from build123d import *

# Parameters (mm, degrees)
F1_W     = 940
F1_H     = 760
F1_W_2   = 30
F1_H_2   = 700
F2_DEPTH = 30
F0_R     = 1.4
F0_R_2   = 13
F3_DEPTH = 5
F4_W     = 30
F4_H     = 30
F5_DEPTH = 770


with BuildPart() as f2:
    # F1 (on Top) → F2 (new body)
    with BuildSketch(Plane.XY):
        with Locations((0, -20)):
            Rectangle(F1_W, F1_H)
        Polygon((-440, -370), (-440, 330), (-80, 330), (-50, 330), (50, 330), (80, 330), (440, 330), (440, -370), (80, -370), (50, -370), (-50, -370), (-80, -370), align=None, mode=Mode.SUBTRACT)
        with Locations((-65, -20)):
            Rectangle(F1_W_2, F1_H_2)
        with Locations((65, -20)):
            Rectangle(F1_W_2, F1_H_2)
    extrude(amount=-F2_DEPTH)

    # F0 (on Top) → F3 (join)
    with BuildSketch(Plane.XY):
        with BuildLine():
            Line((-67.5, 150), (-150, 150))
            Line((-150, 150), (-150, -387.5))
            Line((-150, -387.5), (-140, -387.5))
            ThreePointArc((-140, -387.5), (-137.5, -390), (-140, -392.5))
            Line((-140, -392.5), (-150, -392.5))
            Line((-150, -392.5), (-150, -475))
            Line((-150, -475), (-106, -475))
            ThreePointArc((-106, -475), (-93.5, -469), (-81, -475))
            Line((-81, -475), (0, -475))
            Line((0, -475), (81, -475))
            ThreePointArc((81, -475), (93.5, -469), (106, -475))
            Line((106, -475), (150, -475))
            Line((150, -475), (150, -392.5))
            Line((150, -392.5), (140, -392.5))
            ThreePointArc((140, -392.5), (137.5, -390), (140, -387.5))
            Line((140, -387.5), (150, -387.5))
            Line((150, -387.5), (150, 150))
            Line((150, 150), (67.5, 150))
            Line((67.5, 150), (67.5, 140))
            ThreePointArc((67.5, 140), (65, 137.5), (62.5, 140))
            Line((62.5, 140), (62.5, 150))
            Line((62.5, 150), (-62.5, 150))
            Line((-62.5, 150), (-62.5, 140))
            ThreePointArc((-62.5, 140), (-65, 137.5), (-67.5, 140))
            Line((-67.5, 140), (-67.5, 150))
        make_face()
        with Locations((-106, -468)):
            Circle(F0_R, mode=Mode.SUBTRACT)
        with Locations((-81, -468)):
            Circle(F0_R, mode=Mode.SUBTRACT)
        with Locations((81, -468)):
            Circle(F0_R, mode=Mode.SUBTRACT)
        with Locations((106, -468)):
            Circle(F0_R, mode=Mode.SUBTRACT)
        with Locations((-114.904852, -139.653589)):
            Circle(F0_R, mode=Mode.SUBTRACT)
        with Locations((-139.653589, -114.904852)):
            Circle(F0_R, mode=Mode.SUBTRACT)
        with Locations((-139.653589, 114.904852)):
            Circle(F0_R, mode=Mode.SUBTRACT)
        with Locations((-114.904852, 139.653589)):
            Circle(F0_R, mode=Mode.SUBTRACT)
        with Locations((0, -22)):
            Circle(F0_R, mode=Mode.SUBTRACT)
        with Locations((114.904852, -139.653589)):
            Circle(F0_R, mode=Mode.SUBTRACT)
        with Locations((139.653589, -114.904852)):
            Circle(F0_R, mode=Mode.SUBTRACT)
        Circle(F0_R_2, mode=Mode.SUBTRACT)
        with Locations((0, 22)):
            Circle(F0_R, mode=Mode.SUBTRACT)
        with Locations((114.904852, 139.653589)):
            Circle(F0_R, mode=Mode.SUBTRACT)
        with Locations((139.653589, 114.904852)):
            Circle(F0_R, mode=Mode.SUBTRACT)
    extrude(amount=F3_DEPTH)

    # F4 (on face) → F5 (join)
    with BuildSketch(Plane(origin=(0, 0, -30), x_dir=(1, 0, 0), z_dir=(0, 0, -1))):
        with Locations((-455, 385)):
            Rectangle(F4_W, F4_H)
        with Locations((-455, -345)):
            Rectangle(F4_W, F4_H)
        with Locations((455, -345)):
            Rectangle(F4_W, F4_H)
        with Locations((455, 385)):
            Rectangle(F4_W, F4_H)
    extrude(amount=F5_DEPTH)


solid = f2.part
The listing builds one solid part. Answer for the finished solid, in the listing's coordinates (mm). A direction names the side the tool comes from. Round coordinates to 2 decimals unless told otherwise and drop trailing zeros. Order: outer loops, then holes, each group sorted by start corner. A loop starts at its lowest first (then second) coordinate and runs counter-clockwise, first axis right, second up. Notation, with made-up numbers: (-37, 83) -> (-26, 83) arc R17 ccw to (-26, 97) -> close; hole circle Ø2 at (67.5, 89.25). An arc over 180 degrees is marked (long way). Put each result on its own line as item: value.
Q1. Consider line 1 along Y through (x, z) = (0, 3.95); line 2 along X through (y, z) = (-468, 2.1); line 3 along X through (y, z) = (-393.5, -236). Determine where each line is inside the solid, lowest interval first.
Results list:
line 1: -475 to -23.4, -20.6 to -13, 13 to 20.6, 23.4 to 150
line 2: -150 to -107.4, -104.6 to -82.4, -79.6 to 79.6, 82.4 to 104.6, 107.4 to 150
line 3: -470 to -440, 440 to 470
Q2. Section A-A, the plane y = 44 is taken. Write down the section's boundary in (x, z).
Results list:
outline: (-470, -30) -> (-440, -30) -> (-440, 0) -> (-470, 0) -> close; (-150, 0) -> (-80, 0) -> (-80, -30) -> (-50, -30) -> (-50, 0) -> (50, 0) -> (50, -30) -> (80, -30) -> (80, 0) -> (150, 0) -> (150, 5) -> (-150, 5) -> close; (440, -30) -> (470, -30) -> (470, 0) -> (440, 0) -> close
Q3. Section D-D, the plane y = 273.5 is taken. Write down the section's boundary in (x, z).
Results list:
outline: (-470, -30) -> (-440, -30) -> (-440, 0) -> (-470, 0) -> close; (-80, -30) -> (-50, -30) -> (-50, 0) -> (-80, 0) -> close; (50, -30) -> (80, -30) -> (80, 0) -> (50, 0) -> close; (440, -30) -> (470, -30) -> (470, 0) -> (440, 0) -> close
Q4. Determine the mould class of faces 4 (the flat face through (-2, -400, -13)), 5 (the flat face through (-455, -370, -410)), 6 (the flat face through (-455, -385, -800)), 7 (the flat face through (263, -370, -15)) for opening direction Y: pulls with the +Y half, pulls with the -Y half, needs draft (parallel to the pull), parting line crosses it, or undercut.
Results list:
face 4: pulls with the -Y half
face 5: undercut
face 6: needs draft
face 7: undercut
Q5. Each of these flat-tipped pins is pushed along its axis until it touches: P1, Ø3, axis at x = -139.65, y = 114.9, coming from the -Z side; P2, Ø9, axis at x = 20, z = -16.5, coming from the -Y side; P3, Ø5.5, axis at y = -422.5, z = 3, coming from the -X side. Where does it stop, or does it pass through?
Results list:
P1: z = 0
P2: y = -400
P3: x = -150
Q6. Section C-C, the plane z = -296 is taken. Write down the section's boundary in (x, y), and give its area (3 significant figures).
Results list:
outline: (-470, -400) -> (-440, -400) -> (-440, -370) -> (-470, -370) -> close; (-470, 330) -> (-440, 330) -> (-440, 360) -> (-470, 360) -> close; (440, -400) -> (470, -400) -> (470, -370) -> (440, -370) -> close; (440, 330) -> (470, 330) -> (470, 360) -> (440, 360) -> close
area: 3,600 mm^2
Q7. Section B-B, the plane x = -228 is taken. Write down the section's boundary in (y, z).
Results list:
outline: (-400, -30) -> (-370, -30) -> (-370, 0) -> (-400, 0) -> close; (330, -30) -> (360, -30) -> (360, 0) -> (330, 0) -> close
Q8. Which of the six approach directions +Z, -Z, +X, -X, +Y, -Y give full straight-line access (tool end or side, diameter ignored) to faces 1 (the flat face through (50, -25, -15)), 2 (the flat face through (-263, 330, -15)), 3 (the flat face through (455, 330, -410))?
Results list:
face 1: -Z
face 2: +Z, -Z
face 3: -Z, +X, -X
